Geometry check sheet. Reference: the model listing, model coordinates, mm. Round coordinates to 2 decimals unless told otherwise and drop trailing zeros. Order: outer loops, then holes, each group sorted by start corner. A loop starts at its lowest first (then second) coordinate and runs counter-clockwise, first axis right, second up.
(1) Gauge pin test, flat ends, axial feed: P1, Ø2, axis at x = -26, y = 2.5, coming from the -Z side; P2, Ø3, axis at y = 1.5, z = -35.5, coming from the +X side; P3, Ø1, axis at x = 32, y = 4, coming from the -Z side; P4, Ø12, axis at x = 12.5, z = 35, coming from the +Y side. Record the tip position at first contact, or that the pin passes through.
(2) Cross-section at B-B on x = 0. Enter the section's corners in (y, z) (3 decimals).
(3) Cross-section at D-D on x = -40. Enter the section's corners in (y, z), and give its area (3 significant figures).
(4) Thickness scan on L1, parallel to Z at x = 0, y = 3.95 (3 decimals); L2, parallel to X at y = 5.1, z = -3.5; L3, parallel to X at y = 1.7, z = -18. Record the ranges inside material, lowest first.
(5) Cross-section at A-A on z = 0. Enter the section's corners in (x, y) (3 decimals).
(6) Cross-section at C-C on y = 4.3. Count the separate pieces of the cut face and the enclosed holes in it, and give its area (3 significant figures).
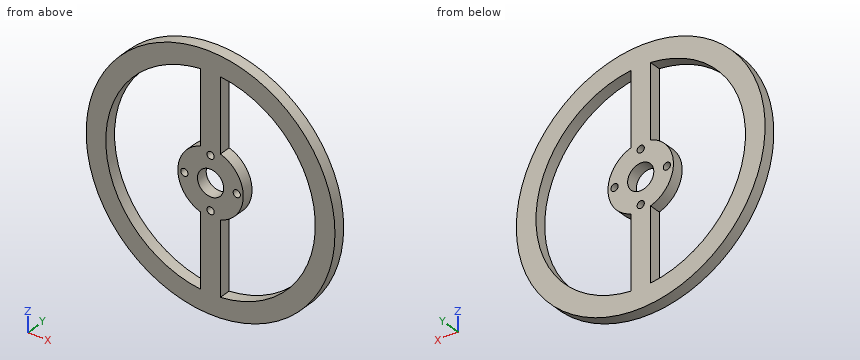
Autodesk Inventor part; units mm, degrees
ref_plane "YZ Plane" through (0, 0, 0) normal (1, 0, 0) x (0, 1, 0)
ref_plane "XZ Plane" through (0, 0, 0) normal (0, 1, 0) x (-1, 0, 0)
ref_plane "XY Plane" through (0, 0, 0) normal (0, 0, 1) x (1, 0, 0)
sketch "Sketch1" plane through (0, 0, 0) normal (0, 1, 0) x (-1, 0, 0)
  circle A0 centre (0, 0) radius 63.5
  circle A1 centre (0, 0) radius 6.35
  circle A2 centre (-12.7, 0) radius 1.75
  circle A3 centre (0, -12.7) radius 1.75
  circle A4 centre (12.7, 0) radius 1.75
  circle A5 centre (0, 12.7) radius 1.75
  dimension "d8" = 3.5
  dimension "d9" = 3.5
  dimension "d10" = 3.5
  dimension "d11" = 3.5
extrude "Extrusion1" add sketch "Sketch1" along normal blind 5.588
sketch "Sketch2" plane through (0, 5.588, 0) normal (0, 1, 0) x (1, 0, 0)
  circle A0 centre (0, 0) radius 63.5
  line L0 (-4.7625, 37.8012) -> (-4.7625, 15.1438)
  line L1 (-4.7625, -15.1438) -> (-4.7625, -37.8012)
  line L2 (4.7625, 37.8012) -> (4.7625, 15.1438)
  line L3 (4.7625, -15.1438) -> (4.7625, -37.8012)
  arc A1 (-4.7625, 15.1438) -> (-4.7625, -15.1438) centre (0, 0) ccw
  arc A2 (4.7625, -15.1438) -> (4.7625, 15.1438) centre (0, 0) ccw
  arc A3 (-4.7625, 50.5763) -> (-4.7625, -50.5763) centre (0, 0) ccw
  arc A4 (4.7625, -50.5763) -> (4.7625, 50.5763) centre (0, 0) ccw
  line L4 (-4.7625, 50.5763) -> (-4.7625, 15.1438)
  line L5 (-4.7625, -15.1438) -> (-4.7625, -50.5763)
  line L6 (4.7625, -50.5763) -> (4.7625, -15.1438)
  line L7 (4.7625, 15.1438) -> (4.7625, 50.5763)
extrude "Extrusion3" cut sketch "Sketch2" against normal blind 25.4 contours L0 A1 L1 L5 A3 L4 | L7 A4 L6 L3 A2 L2
sketch "Sketch3" plane through (0, 5.588, 0) normal (0, 1, 0) x (1, 0, 0)
  circle A0 centre (0, 0) radius 63.5
  circle A1 centre (0, 0) radius 60.325
  dimension "d24" = 120.65
extrude "Extrusion4" cut sketch "Sketch3" against normal blind 25.4
properties part number "AcrylicFlywheel3"
Found:
1. P1: stops at z = -54.9
1. P2: stops at x = 49.83
1. P3: stops at z = -51.45
1. P4: passes through
2. outline: (0, -60.325) - (5.588, -60.325) - (5.588, -14.45) - (0, -14.45) - close; (0, -10.95) - (5.588, -10.95) - (5.588, -6.35) - (0, -6.35) - close; (0, 6.35) - (5.588, 6.35) - (5.588, 10.95) - (0, 10.95) - close; (0, 14.45) - (5.588, 14.45) - (5.588, 60.325) - (0, 60.325) - close
3. outline: (0, -45.16) - (5.59, -45.16) - (5.59, -31.32) - (0, -31.32) - close; (0, 31.32) - (5.59, 31.32) - (5.59, 45.16) - (0, 45.16) - close
3. area: 155 mm2
4. L1: z = -60.325 to -14.45, -10.95 to -6.35, 6.35 to 10.95, 14.45 to 60.325
4. L2: x = -60.22 to -50.68, -15.48 to -5.3, 5.3 to 15.48, 50.68 to 60.22
4. L3: x = -57.58 to -47.5, -4.76 to 4.76, 47.5 to 57.58
5. outline: (-60.325, 0) - (-50.8, 0) - (-50.8, 5.588) - (-60.325, 5.588) - close; (-15.875, 0) - (-14.45, 0) - (-14.45, 5.588) - (-15.875, 5.588) - close; (-10.95, 0) - (-6.35, 0) - (-6.35, 5.588) - (-10.95, 5.588) - close; (6.35, 0) - (10.95, 0) - (10.95, 5.588) - (6.35, 5.588) - close; (14.45, 0) - (15.875, 0) - (15.875, 5.588) - (14.45, 5.588) - close; (50.8, 0) - (60.325, 0) - (60.325, 5.588) - (50.8, 5.588) - close
6. separate pieces: 1
6. enclosed holes: 7
6. area: 4,620 mm2
